Input: part model. Units: mm. Frame: model coordinates. Coordinates: 2 decimals unless noted, no trailing zeros. Loops run counter-clockwise (first coordinate to the right, second up) from the corner with the lowest first, then second, coordinate; pieces in that order, holes last.
(1) Section A-A, the plane x = 175.5. Return loops of the section in (y, z), then the cut area to 3 significant figures.
(2) Contact query for flat-ended pins moving along their axis: P1, Ø8.5, axis at x = 320, z = -215, coming from the +Y side; P2, Ø2.5, axis at x = 61, z = -260, coming from the -Y side. Output: stop coordinate, or through.
(3) Section B-B, the plane z = -313. Return loops of the section in (x, y).
(4) Mould query, pull axis Z, two halves, no side actions, for faces 1 (the face through (326.99, 1.52, -2.85)), 2 (the face through (327.15, 1.52, -276.99)), 3 (the face through (130.925, 1.479, -184.44)). Classes: released by +Z, released by -Z, zero draft, split by the parting line, or undercut.
(5) Section C-C, the plane y = 2.4. Give the number of separate pieces and of enclosed holes in the cut face, then the cut area to 3 significant figures.
(6) Line query: L1, parallel to X at y = 2.3, z = -140; L2, parallel to Z at x = 269, y = 1.75; L3, parallel to Z at x = 165.5, y = 2.75. Output: solid intervals per line, ascending.
(7) Section D-D, the plane x = 45.5. Return loops of the section in (y, z), then the cut area to 3 significant figures.
```python
from build123d import *

# Parameters (mm, degrees)
SKETCH1_W           = 330
SKETCH1_H           = 280
SKETCH1_R           = 56
SKETCH1_W_2         = 190
SKETCH1_H_2         = 70
BOSS_EXTRUDE1_DEPTH = 3
FILLET1_R           = 10
SKETCH2_R           = 2.6
SKETCH2_R_2         = 1.6
CUT_EXTRUDE1_DEPTH  = 482.049893462


with BuildPart() as part:
    # Sketch1 → Boss-Extrude1 (new body)
    # profile 1 of 2: a face of its own
    with BuildSketch(Plane(origin=(0, 0, 0), x_dir=(1, 0, 0), z_dir=(0, 1, 0))):
        with Locations((165, 140)):
            Rectangle(SKETCH1_W, SKETCH1_H)
        with Locations(Location((165, 140, 0), (0, 0, 270))):
            Circle(SKETCH1_R, mode=Mode.SUBTRACT)
    # profile 2 of 2: a face of its own
    with BuildSketch(Plane(origin=(0, 0, 0), x_dir=(1, 0, 0), z_dir=(0, 1, 0))):
        with Locations((165, 315)):
            Rectangle(SKETCH1_W_2, SKETCH1_H_2)
    extrude(amount=BOSS_EXTRUDE1_DEPTH)

    # Fillet1
    fillet1_edges = [part.edges().sort_by_distance(p)[0] for p in [
        (0, 1.5, 0),
        (0, 1.5, -280),
        (70, 1.5, -280),
        (70, 1.5, -350),
        (260, 1.5, -350),
        (260, 1.5, -280),
        (330, 1.5, -280),
        (330, 1.5, 0),
    ]]
    fillet(fillet1_edges, radius=FILLET1_R)

    # Sketch2 → Cut-Extrude1 (cut, through all)
    with BuildSketch(Plane(origin=(0, 3, 0), x_dir=(1, 0, 0), z_dir=(0, 1, 0))):
        with Locations(Location((100, 340, 0), (0, 0, 270))):
            Circle(SKETCH2_R)
        with Locations(Location((230, 340, 0), (0, 0, 270))):
            Circle(SKETCH2_R)
        with Locations(Location((320, 250, 0), (0, 0, 270))):
            Circle(SKETCH2_R)
        with Locations(Location((320, 70, 0), (0, 0, 270))):
            Circle(SKETCH2_R)
        with Locations(Location((260, 10, 0), (0, 0, 270))):
            Circle(SKETCH2_R)
        with Locations(Location((10, 70, 0), (0, 0, 270))):
            Circle(SKETCH2_R)
        with Locations(Location((70, 10, 0), (0, 0, 270))):
            Circle(SKETCH2_R)
        with Locations(Location((10, 250, 0), (0, 0, 270))):
            Circle(SKETCH2_R)
        with Locations(Location((165, 202, 0), (0, 0, 270))):
            Circle(SKETCH2_R_2)
        with Locations(Location((208.840620434, 183.840620434, 0), (0, 0, 270))):
            Circle(SKETCH2_R_2)
        with Locations(Location((227, 140, 0), (0, 0, 270))):
            Circle(SKETCH2_R_2)
        with Locations(Location((208.840620434, 96.159379566, 0), (0, 0, 270))):
            Circle(SKETCH2_R_2)
        with Locations(Location((165, 78, 0), (0, 0, 270))):
            Circle(SKETCH2_R_2)
        with Locations(Location((121.159379566, 96.159379566, 0), (0, 0, 270))):
            Circle(SKETCH2_R_2)
        with Locations(Location((103, 140, 0), (0, 0, 270))):
            Circle(SKETCH2_R_2)
        with Locations(Location((121.159379566, 183.840620434, 0), (0, 0, 270))):
            Circle(SKETCH2_R_2)
        with Locations(Location((35, 260, 0), (0, 0, 270))):
            Circle(SKETCH2_R_2)
        with Locations(Location((61, 260, 0), (0, 0, 270))):
            Circle(SKETCH2_R_2)
        with Locations(Location((87, 260, 0), (0, 0, 270))):
            Circle(SKETCH2_R_2)
        with Locations(Location((113, 260, 0), (0, 0, 270))):
            Circle(SKETCH2_R_2)
        with Locations(Location((139, 260, 0), (0, 0, 270))):
            Circle(SKETCH2_R_2)
        with Locations(Location((165, 260, 0), (0, 0, 270))):
            Circle(SKETCH2_R_2)
        with Locations(Location((191, 260, 0), (0, 0, 270))):
            Circle(SKETCH2_R_2)
        with Locations(Location((217, 260, 0), (0, 0, 270))):
            Circle(SKETCH2_R_2)
        with Locations(Location((243, 260, 0), (0, 0, 270))):
            Circle(SKETCH2_R_2)
        with Locations(Location((269, 260, 0), (0, 0, 270))):
            Circle(SKETCH2_R_2)
        with Locations(Location((295, 260, 0), (0, 0, 270))):
            Circle(SKETCH2_R_2)
        with Locations(Location((35, 40, 0), (0, 0, 270))):
            Circle(SKETCH2_R_2)
        with Locations(Location((61, 40, 0), (0, 0, 270))):
            Circle(SKETCH2_R_2)
        with Locations(Location((87, 40, 0), (0, 0, 270))):
            Circle(SKETCH2_R_2)
        with Locations(Location((113, 40, 0), (0, 0, 270))):
            Circle(SKETCH2_R_2)
        with Locations(Location((139, 40, 0), (0, 0, 270))):
            Circle(SKETCH2_R_2)
        with Locations(Location((165, 40, 0), (0, 0, 270))):
            Circle(SKETCH2_R_2)
        with Locations(Location((191, 40, 0), (0, 0, 270))):
            Circle(SKETCH2_R_2)
        with Locations(Location((217, 40, 0), (0, 0, 270))):
            Circle(SKETCH2_R_2)
        with Locations(Location((243, 40, 0), (0, 0, 270))):
            Circle(SKETCH2_R_2)
        with Locations(Location((269, 40, 0), (0, 0, 270))):
            Circle(SKETCH2_R_2)
        with Locations(Location((295, 40, 0), (0, 0, 270))):
            Circle(SKETCH2_R_2)
        with Locations(Location((10, 215, 0), (0, 0, 270))):
            Circle(SKETCH2_R)
        with Locations(Location((10, 105, 0), (0, 0, 270))):
            Circle(SKETCH2_R)
        with Locations(Location((105, 10, 0), (0, 0, 270))):
            Circle(SKETCH2_R)
        with Locations(Location((225, 10, 0), (0, 0, 270))):
            Circle(SKETCH2_R)
        with Locations(Location((320, 105, 0), (0, 0, 270))):
            Circle(SKETCH2_R)
        with Locations(Location((320, 215, 0), (0, 0, 270))):
            Circle(SKETCH2_R)
        with Locations(Location((135, 340, 0), (0, 0, 270))):
            Circle(SKETCH2_R)
        with Locations(Location((195, 340, 0), (0, 0, 270))):
            Circle(SKETCH2_R)
    extrude(amount=-CUT_EXTRUDE1_DEPTH, mode=Mode.SUBTRACT)


solid = part.part
```
Report:
1. outline: (0, -350) - (3, -350) - (3, -195.01) - (0, -195.01) - close; (0, -84.99) - (3, -84.99) - (3, 0) - (0, 0) - close
1. area: 720 mm2
2. P1: stops at y = 3
2. P2: passes through
3. outline: (70, 0) - (260, 0) - (260, 3) - (70, 3) - close
4. face 1: released by +Z
4. face 2: released by -Z
4. face 3: undercut
5. separate pieces: 1
5. enclosed holes: 47
5. area: 95,200 mm2
6. L1: x = 0 to 101.4, 104.6 to 109, 221 to 225.4, 228.6 to 330
6. L2: z = -280.05 to -261.6, -258.4 to -41.6, -38.4 to 0
6. L3: z = -350 to -261.52, -258.48 to -203.52, -200.48 to -196, -84 to -79.52, -76.48 to -41.52, -38.48 to 0
7. outline: (0, -280) - (3, -280) - (3, 0) - (0, 0) - close
7. area: 840 mm2
